Design review of the part built by this model. Coordinates are the model's own, in mm. Give positions to 0.01 mm unless a question says otherwise; leave off trailing zeros. Write each loop counter-clockwise with the first axis right and the second up, starting at its lowest first coordinate (ties: lowest second). Pieces come first, ordered by that corner, then holes. Notation, with made-up numbers: M 49.5,17.5 L 78.5,17.5 A23 ccw 78.5,31.5 Z; hole C 25.25,65 d11. An arc over 180 degrees is marked long. Use a Markdown table: item, result. Add a question column.
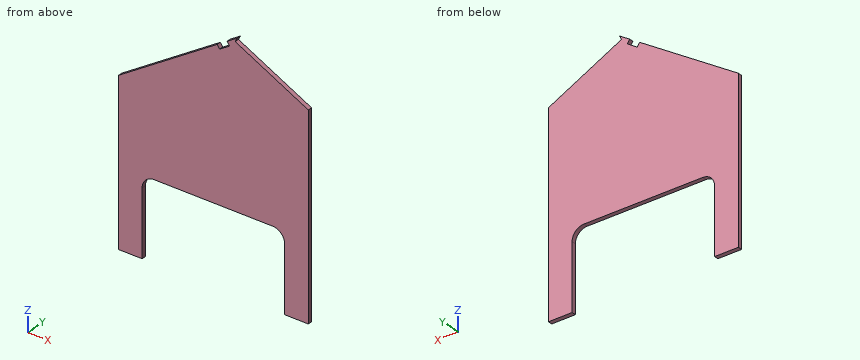
```python
from build123d import *

# Parameters (mm, degrees)
F1_DEPTH = 18
F5_DEPTH = 18
F7_DEPTH = 18


with BuildPart() as f1:
    # F0 (on Front) → F1 (new body)
    with BuildSketch(Plane.XZ):
        with BuildLine():
            Line((0, 675), (0, 0))
            Line((0, 0), (100, 0))
            Line((100, 0), (100, 275))
            ThreePointArc((100, 275), (114.644661, 310.355339), (150, 325))
            Line((150, 325), (650, 325))
            ThreePointArc((650, 325), (685.355339, 310.355339), (700, 275))
            Line((700, 275), (700, 0))
            Line((700, 0), (800, 0))
            Line((800, 0), (800, 850))
            Line((800, 850), (500, 1000))
            Line((500, 1000), (0, 675))
        make_face()
    extrude(amount=F1_DEPTH)

    # F4 (on face) → F5 (cut)
    with BuildSketch(Plane.XZ.offset(18)):
        Polygon((458.077819, 972.750582), (416.155638, 945.501165), (425.965429, 930.40918), (467.887609, 957.658597), align=None)
    extrude(amount=-F5_DEPTH, mode=Mode.SUBTRACT)

    # F6 (on face) → F7 (cut, through all)
    with BuildSketch(Plane.XZ.offset(18)):
        Polygon((500, 1000), (491.950155, 983.900311), (849.721032, 805.014872), (857.770876, 821.114562), align=None)
    extrude(amount=-F7_DEPTH, mode=Mode.SUBTRACT)


solid = f1.part
```
(1) Wall thickness on L1, parallel to X at y = -15, z = 240.5; L2, parallel to X at y = -10, z = 939; L3, parallel to Z at x = 444, y = -6.5: over which ranges is each line inside the solid? List them lowest first.
(2) Add section C-C on z = 720. Give the boundary of the cut face in (x, y).
(3) For pin 1 (4 mm diameter, centred on x = 202.5, y = -9, fed in from +Z) (3 decimals); pin 2 (5 mm diameter, centred on x = 238.5, y = -5.5, fed in from +Z); pin 3 (6 mm diameter, centred on y = -6.5, z = 845, fed in from +X), all flat-tipped, find the tip position at first contact; note any pin that passes through.
(4) Add section A-A on y = -11.5. Give the boundary of the cut face in (x, z).
(5) Add section B-B on x = 259. Give the boundary of the cut face in (y, z), then the cut area to 3 significant figures.
From the geometry:
| question | item | result |
|---|---|---|
| 1 | L1 | x = 0 to 100, 700 to 800 |
| 1 | L2 | x = 406.15 to 420.38, 439.18 to 581.75 |
| 1 | L3 | z = 325 to 942.13 |
| 2 | outline | M 69.23,-18 L 800,-18 L 800,0 L 69.23,0 Z |
| 3 | pin 1 | stops at z = 807.925 |
| 3 | pin 2 | stops at z = 831.65 |
| 3 | pin 3 | stops at x = 775.75 |
| 4 | outline | M 0,0 L 100,0 L 100,275 A50 cw 150,325 L 650,325 A50 cw 700,275 L 700,0 L 800,0 L 800,829.88 L 491.95,983.9 L 425.97,930.41 L 416.16,945.5 L 0,675 Z |
| 5 | outline | M -18,325 L 0,325 L 0,843.35 L -18,843.35 Z |
| 5 | area | 9,330 mm^2 |
